Could you check a few things on this model? Use its own coordinates, in mm. A direction names the side the tool comes from. Give positions to 0.01 mm unless a question says otherwise; leave off trailing zeros. Order: outer loops, then holes, each group sorted by start corner. A loop starts at its lowest first (then second) coordinate and runs counter-clockwise, first axis right, second up.
(1) On a 3-axis mill with a long thin cutter (end or side, diameter ignored), from which of +Z, -Z, +X, -X, +Y, -Y can I reach the whole of each face in a straight line? I mean faces 4 (the cylindrical face through (-15.914, -0.493, -4.208)), 5 (the flat face through (0, 0, 0)). Say none if no direction works.
(2) Will these pins go through, and if not, where does the flat tip stop? pin 1 (2.5 mm diameter, centred on x = 11.5, y = 7, fed in from -Z); pin 2 (1 mm diameter, centred on x = 12.5, z = 17.5, fed in from -Y); pin 3 (5 mm diameter, centred on x = -11.5, y = 30, fed in from -Z); pin 4 (11 mm diameter, centred on x = 3.5, z = 2, fed in from +Y).
(3) Imagine slicing it at D-D, the plane z = -4. Write out the boundary of the cut face in (x, y), then the cut area to 3 significant figures.
(4) Imagine slicing it at C-C, the plane x = -11.5. Write out the boundary of the cut face in (y, z), then the cut area to 3 significant figures.
(5) If I drill on probe 1 along X at (y, z) = (-0.7, 7.5); probe 2 along Y at (x, z) = (-11.5, 21.25); probe 3 along X at (y, z) = (14, 21), over which ranges is the centre line in solid material (lowest first)?
(6) If we mould it in two halves opening along X, with no side actions, what happens to faces 1 (the cylindrical face through (-10.27, 6.06, 21.36)), 2 (the flat face through (25, 8.8, 21.2)), 3 (the cylindrical face through (-24.43, 35.29, 21.36))? For each: released by +X, released by -X, zero draft, split by the parting line, or undercut.
(7) Imagine slicing it at B-B, the plane y = 30. Write out the boundary of the cut face in (x, z), then the cut area to 3 significant figures.
(8) Imagine slicing it at A-A, the plane y = 26. Write out the boundary of the cut face in (x, z).
from build123d import *

# Parameters (mm, degrees)
SKETCH_1_W                       = 50
SKETCH_1_H                       = 22
SKETCH_1_R                       = 1.6
SM_BASE_FLANGE_1_DEPTH           = 1
SM_EDGE_FLANGE_5_STRIP_CUT_DEPTH = 50
SM_EDGE_FLANGE_5_DEPTH           = 50
SM_EDGE_FLANGE_4_STRIP_CUT_DEPTH = 50
SM_EDGE_FLANGE_4_DEPTH           = 50
SKETCH_9_R                       = 1.55
SKETCH_9_R_2                     = 1.05
SKETCH_9_R_3                     = 6.05
SKETCH_9_R_4                     = 4.1
CUT_EXTRUDE_1_DEPTH              = 10
FILLET_1_R                       = 2


# Sheet-metal steps are written as plain solids
with BuildPart() as part:
    # Sketch 1 → 基体-法兰1 (new body)
    with BuildSketch(Plane(origin=(0, 0, 0), x_dir=(1, 0, 0), z_dir=(0, 1, 0))):
        Rectangle(SKETCH_1_W, SKETCH_1_H)
        with Locations(Location((0, -7.5, 0), (0, 0, 270))):
            Circle(SKETCH_1_R, mode=Mode.SUBTRACT)
        with Locations(Location((-17.5, 4, 0), (0, 0, 270))):
            Circle(SKETCH_1_R, mode=Mode.SUBTRACT)
        with Locations(Location((17.5, 4, 0), (0, 0, 90))):
            Circle(SKETCH_1_R, mode=Mode.SUBTRACT)
    extrude(amount=-SM_BASE_FLANGE_1_DEPTH)

    # 边线-法兰5 strip (across the edge) → 边线-法兰5 strip cut (cut)
    with BuildSketch(Plane(origin=(-25, 0, 11), x_dir=(0, 0.9396926207859105, -0.3420201433256631), z_dir=(1, 0, 0))):
        Polygon((-2.767214854, 4.679055925), (-0.895270205, -0.464069727), (0.044422416, -0.122049584), (-1.827522233, 5.021076069), align=None)
    extrude(amount=SM_EDGE_FLANGE_5_STRIP_CUT_DEPTH, mode=Mode.SUBTRACT)

    # 边线-法兰5 section (across the edge) → 边线-法兰5 (add)
    with BuildSketch(Plane(origin=(-25, 0, 11), x_dir=(0, 0.9396926207859105, -0.3420201433256631), z_dir=(1, 0, 0))):
        with BuildLine():
            Line((-1, 0.129882454), (-1, 10.5))
            Line((-1, 10.5), (0, 10.5))
            Line((0, 10.5), (0, 0.129882454))
            ThreePointArc((0, 0.129882454), (0.011190609, 0.001973206), (0.044422416, -0.122049584))
            Line((0.044422416, -0.122049584), (-0.895270205, -0.464069727))
            ThreePointArc((-0.895270205, -0.464069727), (-0.973617144, -0.171674971), (-1, 0.129882454))
        make_face()
    extrude(amount=SM_EDGE_FLANGE_5_DEPTH)

    # 边线-法兰4 strip (across the edge) → 边线-法兰4 strip cut (cut)
    with BuildSketch(Plane(origin=(-25, 3.591211505, 20.866772518), x_dir=(0, 0, -1), z_dir=(1, 0, 0))):
        Polygon((-5.000477833, 0.755847316), (0.142647819, -1.116097333), (0.484667962, -0.176404712), (-4.65845769, 1.695539937), align=None)
    extrude(amount=SM_EDGE_FLANGE_4_STRIP_CUT_DEPTH, mode=Mode.SUBTRACT)

    # 边线-法兰4 section (across the edge) → 边线-法兰4 (add)
    with BuildSketch(Plane(origin=(-25, 3.591211505, 20.866772518), x_dir=(0, 0, -1), z_dir=(1, 0, 0))):
        with BuildLine():
            Line((-1, 0.515772873), (-1, 32.299792462))
            Line((-1, 32.299792462), (0, 32.299792462))
            Line((0, 32.299792462), (0, 0.515772873))
            ThreePointArc((0, 0.515772873), (0.133212604, 0.09327647), (0.484667962, -0.176404712))
            Line((0.484667962, -0.176404712), (0.142647819, -1.116097333))
            ThreePointArc((0.142647819, -1.116097333), (-0.68593944, -0.480299967), (-1, 0.515772873))
        make_face()
    extrude(amount=SM_EDGE_FLANGE_4_DEPTH)

    # 草图9 → 切除-拉伸1 (cut)
    # profile 1 of 12: a face of its own
    with BuildSketch(Plane(origin=(0, 0, 20.866772518), x_dir=(-1, 0, 0), z_dir=(0, 0, -1))):
        with Locations((-11.5, 30)):
            Circle(SKETCH_9_R)
    # profile 2 of 12: a face of its own
    with BuildSketch(Plane(origin=(0, 0, 20.866772518), x_dir=(-1, 0, 0), z_dir=(0, 0, -1))):
        with Locations((11.5, 30)):
            Circle(SKETCH_9_R)
    # profile 3 of 12: a face of its own
    with BuildSketch(Plane(origin=(0, 0, 20.866772518), x_dir=(-1, 0, 0), z_dir=(0, 0, -1))):
        with Locations((6.495190528, 22.25)):
            Circle(SKETCH_9_R_2)
    # profile 4 of 12: a face of its own
    with BuildSketch(Plane(origin=(0, 0, 20.866772518), x_dir=(-1, 0, 0), z_dir=(0, 0, -1))):
        with Locations((0, 26)):
            Circle(SKETCH_9_R_2)
    # profile 5 of 12: a face of its own
    with BuildSketch(Plane(origin=(0, 0, 20.866772518), x_dir=(-1, 0, 0), z_dir=(0, 0, -1))):
        with Locations((-6.495190528, 22.25)):
            Circle(SKETCH_9_R_2)
    # profile 6 of 12: a face of its own
    with BuildSketch(Plane(origin=(0, 0, 20.866772518), x_dir=(-1, 0, 0), z_dir=(0, 0, -1))):
        with Locations((-6.495190528, 14.75)):
            Circle(SKETCH_9_R_2)
    # profile 7 of 12: a face of its own
    with BuildSketch(Plane(origin=(0, 0, 20.866772518), x_dir=(-1, 0, 0), z_dir=(0, 0, -1))):
        with Locations((0, 11)):
            Circle(SKETCH_9_R_2)
    # profile 8 of 12: a face of its own
    with BuildSketch(Plane(origin=(0, 0, 20.866772518), x_dir=(-1, 0, 0), z_dir=(0, 0, -1))):
        with Locations((6.495190528, 14.75)):
            Circle(SKETCH_9_R_2)
    # profile 9 of 12: a face of its own
    with BuildSketch(Plane(origin=(0, 0, 20.866772518), x_dir=(-1, 0, 0), z_dir=(0, 0, -1))):
        with Locations((0, 18.5)):
            Circle(SKETCH_9_R_3)
        with Locations((0, 18.5)):
            Circle(SKETCH_9_R_4, mode=Mode.SUBTRACT)
    # profile 10 of 12: a face of its own
    with BuildSketch(Plane(origin=(0, 0, 20.866772518), x_dir=(-1, 0, 0), z_dir=(0, 0, -1))):
        with Locations((0, 18.5)):
            Circle(SKETCH_9_R_4)
    # profile 11 of 12: a face of its own
    with BuildSketch(Plane(origin=(0, 0, 20.866772518), x_dir=(-1, 0, 0), z_dir=(0, 0, -1))):
        with Locations((11.5, 7)):
            Circle(SKETCH_9_R)
    # profile 12 of 12: a face of its own
    with BuildSketch(Plane(origin=(0, 0, 20.866772518), x_dir=(-1, 0, 0), z_dir=(0, 0, -1))):
        with Locations((-11.5, 7)):
            Circle(SKETCH_9_R)
    extrude(amount=-CUT_EXTRUDE_1_DEPTH, mode=Mode.SUBTRACT)

    # 圆角1
    fillet_1_edges = [part.edges().sort_by_distance(p)[0] for p in [
        (-25, 35.891003967, 21.366772518),
        (-25, -0.5, -11),
        (25, -0.5, -11),
        (25, 35.891003967, 21.366772518),
    ]]
    fillet(fillet_1_edges, radius=FILLET_1_R)


solid = part.part
Answer block:
1. face 4: +Y, -Y
1. face 5: -Z, +X, -X, +Y
2. pin 1: passes through
2. pin 2: stops at y = 1.12
2. pin 3: stops at z = 20.87
2. pin 4: stops at y = 0
3. outline: (-25, -1) - (-19.1, -1) - (-19.1, 0) - (-25, 0) - close; (-15.9, -1) - (15.9, -1) - (15.9, 0) - (-15.9, 0) - close; (19.1, -1) - (25, -1) - (25, 0) - (19.1, 0) - close
3. area: 43.6 mm2
4. outline: (-1, -11) - (0, -11) - (0, 10.87) arc R0.74 cw to (0.04, 11.12) - (3.41, 20.38) arc R0.74 cw to (4.11, 20.87) - (5.45, 20.87) - (5.45, 21.87) - (4.11, 21.87) arc R1.74 ccw to (2.48, 20.72) - (-0.9, 11.46) arc R1.74 ccw to (-1, 10.87) - close; (8.55, 20.87) - (28.45, 20.87) - (28.45, 21.87) - (8.55, 21.87) - close; (31.55, 20.87) - (35.89, 20.87) - (35.89, 21.87) - (31.55, 21.87) - close
4. area: 59.3 mm2
5. probe 1: x = -25 to -1.6, 1.6 to 25
5. probe 2: y = 2.78 to 5.45, 8.55 to 28.45, 31.55 to 35.89
5. probe 3: x = -25 to -7.23, -5.76 to -4.04, 4.04 to 5.76, 7.23 to 25
6. face 1: undercut
6. face 2: released by +X
6. face 3: released by -X
7. outline: (-25, 20.87) - (-13.05, 20.87) - (-13.05, 21.87) - (-25, 21.87) - close; (-9.95, 20.87) - (9.95, 20.87) - (9.95, 21.87) - (-9.95, 21.87) - close; (13.05, 20.87) - (25, 20.87) - (25, 21.87) - (13.05, 21.87) - close
7. area: 43.8 mm2
8. outline: (-25, 20.87) - (-1.05, 20.87) - (-1.05, 21.87) - (-25, 21.87) - close; (1.05, 20.87) - (25, 20.87) - (25, 21.87) - (1.05, 21.87) - close
